Input: part model. Units: mm. Frame: model coordinates. A direction names the side the tool comes from. Give positions to 0.01 mm unless a question says otherwise; leave off trailing zeros. Loops run counter-clockwise (first coordinate to the right, second up) from the corner with the lowest first, then second, coordinate; pieces in that order, holes last. Notation, with made-up numbers: (63.5, -17.5) -> (89.5, -17.5) arc R15 cw to (89.5, 2.5) -> close; hole circle Ø9 at (49, 62.5). An arc over 180 degrees is marked (long way). One line per question, with ' | ' between items.
from build123d import *

# Parameters (mm, degrees)
SKETCH1_W           = 233.68
SKETCH1_H           = 233.68
BOSS_EXTRUDE1_DEPTH = 165.1


with BuildPart() as part:
    # Sketch1 → Boss-Extrude1 (new body)
    with BuildSketch(Plane(origin=(0, 0, 0), x_dir=(1, 0, 0), z_dir=(0, 1, 0))):
        Rectangle(SKETCH1_W, SKETCH1_H)
    extrude(amount=BOSS_EXTRUDE1_DEPTH)

    # Sketch3 → Revolve1 (revolve)
    with BuildSketch(Plane.YZ.offset(-43.40946291)):
        with BuildLine():
            Line((165.1, 43.916968586), (309.883452069, 43.916968586))
            ThreePointArc((309.883452069, 43.916968586), (290.37259982, -3.186395526), (243.269235708, -22.697247775))
            Line((243.269235708, -22.697247775), (165.1, -22.697247775))
            Line((165.1, -22.697247775), (165.1, 43.916968586))
        make_face()
    revolve(axis=Axis((-43.40946291, 165.1, 43.916968586), (0, 1, 0)))


solid = part.part
1. Section query B-B (z = 103). Output: boundary loops of the cut face in (x, y).
Determined:
outline: (-116.84, 0) -> (116.84, 0) -> (116.84, 165.1) -> (-12.64, 165.1) -> (-12.64, 243.27) arc R30.77 ccw to (-74.18, 243.27) -> (-74.18, 165.1) -> (-116.84, 165.1) -> close
2. Pin query (flat end, axial travel): P1, Ø2, axis at x = -83, y = 227.5, coming from the +Z side; P2, Ø3, axis at y = 218.5, z = 77, coming from the +X side; P3, Ø10, axis at x = 13.5, y = 214, coming from the -Z side. Return the tip coordinate at first contact, or that it passes through.
Determined:
P1: stops at z = 98.21 | P2: stops at x = 15.24 | P3: stops at z = 2.17
3. Section query D-D (x = 69.5). Output: boundary loops of the cut face in (y, z).
Determined:
outline: (0, -116.84) -> (165.1, -116.84) -> (165.1, 116.84) -> (0, 116.84) -> close
4. Reachability of faces 1 (the cylindrical face through (-63.42, 203.64, -19.62)), 2 (the flat face through (-2, 81, -116.84)) from +Z, -Z, +X, -X, +Y, -Y: full face, straight path, thin tool, end or side. Return the list, or none.
Determined:
face 1: +Y | face 2: -Z, +X, -X, +Y, -Y
5. Section query C-C (y = 268.5). Output: boundary loops of the cut face in (x, z).
Determined:
outline: circle Ø123.3 at (-43.41, 43.92)
6. Section query A-A (x = -30.5). Output: boundary loops of the cut face in (y, z).
Determined:
outline: (0, -116.84) -> (165.1, -116.84) -> (165.1, -21.43) -> (243.27, -21.43) arc R65.35 ccw to (243.27, 109.27) -> (165.1, 109.27) -> (165.1, 116.84) -> (0, 116.84) -> close
7. Ray query, line 1 along Y through (x, z) = (82, -66); line 2 along Z through (x, y) = (-47.5, 239.5); line 3 along Z through (x, y) = (-60, 297.5). Return the intervals inside material, ascending. Write a range as from..to.
Determined:
line 1: y = 0..165.1 | line 2: z = -22.57..110.41 | line 3: z = 8.97..78.86
